from build123d import *

# Parameters (mm, degrees)
SKETCH001_R     = 11
POCKET_DEPTH    = 10
CHAMFER_1_SIZE2 = 0.5
CHAMFER_1_SIZE  = 1
CHAMFER_2_SIZE2 = 0.5
CHAMFER_2_SIZE  = 1
FILLET_R        = 1


with BuildPart() as part:
    # Sketch → Revolution (revolve)
    with BuildSketch(Plane.XY):
        Polygon((0, 0), (-14, 0), (-13, 1.5), (-13, 8.5), (-14, 10), (0, 10), align=None)
    revolve(axis=Axis((0, 0, 0), (0, 1, 0)))

    # Sketch001 (on Face1 of Revolution) → Pocket (cut)
    with BuildSketch(Plane.XZ):
        Circle(SKETCH001_R)
    extrude(amount=-POCKET_DEPTH, mode=Mode.SUBTRACT)

    # Chamfer 1
    chamfer_1_edges = [part.edges().sort_by_distance(p)[0] for p in [
        (-11, 10, 0),
    ]]
    chamfer_1_side = part.faces().sort_by_distance((-11, 5, 0))[0]
    chamfer(chamfer_1_edges, length=CHAMFER_1_SIZE, length2=CHAMFER_1_SIZE2, reference=chamfer_1_side)

    # Chamfer 2
    chamfer_2_edges = [part.edges().sort_by_distance(p)[0] for p in [
        (-11, 0, 0),
    ]]
    chamfer_2_side = part.faces().sort_by_distance((13.60402, 0, 0))[0]
    chamfer(chamfer_2_edges, length=CHAMFER_2_SIZE, length2=CHAMFER_2_SIZE2, reference=chamfer_2_side)

    # Fillet
    fillet_edges = [part.edges().sort_by_distance(p)[0] for p in [
        (-11, 9, 0),
        (-11, 0.5, 0),
    ]]
    fillet(fillet_edges, radius=FILLET_R)


solid = part.part
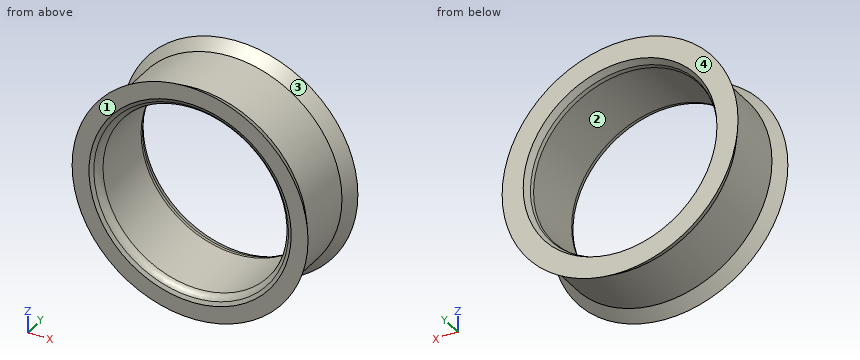
Part model, mm, in its own coordinate system. Face numbers are marked on the shaded views. Round coordinates to 2 decimals unless told otherwise and drop trailing zeros. Write each loop counter-clockwise with the first axis right and the second up, starting at its lowest first coordinate (ties: lowest second). Pieces come first, ordered by that corner, then holes. Notation, with made-up numbers: M -37.5,50.25 L -32.5,50.25 A13 cw -32.5,63.25 Z; hole C 60,-27.5 d1. An arc over 180 degrees is marked long. Return JSON: item names as keys, results as strings. Group by question number.
(1) Two-plate mould, pull along Y, no slides. Class the marked faces 1, 2, 3 and 4: +Y half, -Y half, draft (parallel to the pull), parting line (faces both ways), or undercut.
(2) Pin check, flat tips, straight feed: pin 1 Ø1 at (x, y) = (-10, 4) entering from +Z; pin 2 Ø2 at (x, y) = (-7.5, 2.5) entering from -Z; pin 3 Ø6 at (y, z) = (8.5, 5.5) entering from -X; pin 4 Ø13 at (x, z) = (0, 0) entering from -Y. Stop position of each tip, or through.
(3) Drill centre lines: probe 1 along Z at (x, y) = (0, 4.5); probe 2 along Z at (x, y) = (7.5, 1.5); probe 3 along X at (y, z) = (8, -1.5). Where is each one in solid material? Low to high.
(4) Saw through at A-A on y = 7. Write the cut outline in (x, z), then the cut area to 3 significant figures.
Returned:
{
 "1": {"face 1": "-Y half", "face 2": "draft", "face 3": "undercut", "face 4": "+Y half"},
 "2": {"pin 1": "z = 8.87", "pin 2": "z = -11.26", "pin 3": "x = -13.7", "pin 4": "through"},
 "3": {"probe 1": "-13 to -11, 11 to 13", "probe 2": "-10.62 to -8.05, 8.05 to 10.62", "probe 3": "-12.91 to -10.9, 10.9 to 12.91"},
 "4": {"outline": "C 0,0 d26; hole C 0,0 d22", "area": "151 mm²"}
}
